from build123d import *

# Parameters (mm, degrees)
EXTRUDE_1_DEPTH     = 30
SKETCH_2_W          = 20
SKETCH_2_H          = 30.268482551
CUT_EXTRUDE_1_DEPTH = 27


with BuildPart() as part:
    # 草圖1 → 填料-伸長1 (new body)
    with BuildSketch(Plane.XY):
        Polygon((-18.940316301, 5.568561873), (11.059683699, -39.431438127), (11.059683699, 20.568561873), (-18.940316301, 20.568561873), align=None)
    extrude(amount=EXTRUDE_1_DEPTH)

    # 草圖2 → 除料-伸長1 (cut)
    with BuildSketch(Plane.ZY.offset(18.940316301)):
        with Locations((15, -13.262891615)):
            Rectangle(SKETCH_2_W, SKETCH_2_H)
    extrude(amount=-CUT_EXTRUDE_1_DEPTH, mode=Mode.SUBTRACT)


solid = part.part
CAD build for the part. Positions are in the model's coordinates, mm. A direction names the side the tool comes from. Give positions to 0.01 mm unless a question says otherwise; leave off trailing zeros. Order: outer loops, then holes, each group sorted by start corner. A loop starts at its lowest first (then second) coordinate and runs counter-clockwise, first axis right, second up. Notation, with made-up numbers: (7.25, 9) - (57.25, 9) arc R24 cw to (57.25, 41) - close; hole circle Ø10 at (86.25, -12). An arc over 180 degrees is marked (long way). Answer in a Markdown table with one row per item.
1. Tool access for faces 1 (the flat face through (-1, -2, 0)), 2 (the flat face through (6, -28.397, 15)): list every direction of +Z, -Z, +X, -X, +Y, -Y with a clear straight run to the whole face (end or side of a thin tool).
Data:
| item | result |
|---|---|
| face 1 | -Z, +X, -X, +Y, -Y |
| face 2 | -X |
2. Flat gauge pins, fed straight in: pin 1 (16 mm diameter, centred on y = -18.5, z = 16, fed in from -X); pin 2 (4 mm diameter, centred on y = -7.5, z = 5, fed in from -X). Where does each tip first touch, or does it go through?
Data:
| item | result |
|---|---|
| pin 1 | stops at x = 8.06 |
| pin 2 | stops at x = -11.56 |
3. Pull direction Z, two halves, no side cores. Call faces 3 (the flat face through (-4, 20.569, 15)), 4 (the flat face through (-2, -10, 5)), 5 (the flat face through (-2, -10, 25)), 6 (the flat face through (-1, -2, 30)): pulls with the +Z half, pulls with the -Z half, needs draft (parallel to the pull), parting line crosses it, or undercut.
Data:
| item | result |
|---|---|
| face 3 | needs draft |
| face 4 | undercut |
| face 5 | undercut |
| face 6 | pulls with the +Z half |
4. Probe probe 1 along Z at (x, y) = (-6.75, 1); probe 2 along Y at (x, z) = (-4.25, 2.5); probe 3 along Y at (x, z) = (1.25, 16.25). List the from-to ranges inside material, lowest first. Write a range as [from, to].
Data:
| item | result |
|---|---|
| probe 1 | z = [0, 5], [25, 30] |
| probe 2 | y = [-16.47, 20.57] |
| probe 3 | y = [1.87, 20.57] |
5. Saw through at A-A, the plane z = 21.25. Give the cut face in (x, y), plus the area to 3 significant figures.
Data:
| item | result |
|---|---|
| outline | (-18.94, 5.57) - (-16.48, 1.87) - (8.06, 1.87) - (8.06, -28.4) - (3.7, -28.4) - (11.06, -39.43) - (11.06, 20.57) - (-18.94, 20.57) - close |
| area | 688 mm² |
6. Saw through at B-B, the plane y = -17. Give the cut face in (x, z).
Data:
| item | result |
|---|---|
| outline | (-3.89, 0) - (11.06, 0) - (11.06, 30) - (-3.89, 30) - (-3.89, 25) - (8.06, 25) - (8.06, 5) - (-3.89, 5) - close |
7. Saw through at C-C, the plane z = 25.75. Give the cut face in (x, y), plus the area to 4 significant figures.
Data:
| item | result |
|---|---|
| outline | (-18.94, 5.57) - (11.06, -39.43) - (11.06, 20.57) - (-18.94, 20.57) - close |
| area | 1,125 mm² |
8. Saw through at D-D, the plane y = -33. Give the cut face in (x, z), plus the area to 3 significant figures.
Data:
| item | result |
|---|---|
| outline | (6.77, 0) - (11.06, 0) - (11.06, 30) - (6.77, 30) - close |
| area | 129 mm² |
